```python
from build123d import *

# Parameters (mm, degrees)
SKETCH1_R           = 114.3
SKETCH1_R_2         = 1.778
SKETCH1_W           = 31.75
SKETCH1_H           = 69.85
BOSS_EXTRUDE1_DEPTH = 3.175
SKETCH2_R           = 1.778
SKETCH2_R_2         = 3.914780109
CUT_EXTRUDE1_DEPTH  = 25.4


with BuildPart() as part:
    # Sketch1 → Boss-Extrude1 (new body)
    with BuildSketch(Plane(origin=(0, 0, 0), x_dir=(1, 0, 0), z_dir=(0, 1, 0))):
        Circle(SKETCH1_R)
        with Locations((-14.986, 82.55)):
            Circle(SKETCH1_R_2, mode=Mode.SUBTRACT)
        with Locations((14.986, 82.55)):
            Circle(SKETCH1_R_2, mode=Mode.SUBTRACT)
        with Locations((-14.986, 58.674)):
            Circle(SKETCH1_R_2, mode=Mode.SUBTRACT)
        with Locations((14.986, 58.674)):
            Circle(SKETCH1_R_2, mode=Mode.SUBTRACT)
        with Locations((25.4, 7.874)):
            Circle(SKETCH1_R_2, mode=Mode.SUBTRACT)
        with Locations((25.4, 0)):
            Circle(SKETCH1_R_2, mode=Mode.SUBTRACT)
        with Locations((-25.4, 7.874)):
            Circle(SKETCH1_R_2, mode=Mode.SUBTRACT)
        with Locations((-25.4, 0)):
            Circle(SKETCH1_R_2, mode=Mode.SUBTRACT)
        with Locations((64.389, -15.24)):
            Rectangle(SKETCH1_W, SKETCH1_H, mode=Mode.SUBTRACT)
        with Locations((-64.389, -15.24)):
            Rectangle(SKETCH1_W, SKETCH1_H, mode=Mode.SUBTRACT)
    extrude(amount=BOSS_EXTRUDE1_DEPTH)

    # Sketch2 → Cut-Extrude1 (cut)
    with BuildSketch(Plane(origin=(0, 3.175, 0), x_dir=(1, 0, 0), z_dir=(0, 1, 0))):
        with Locations((-48.514, 32.385)):
            Circle(SKETCH2_R)
        with Locations((48.514, 32.385)):
            Circle(SKETCH2_R)
        with Locations((38.1, 4.739101121)):
            Circle(SKETCH2_R)
        with Locations((-38.1, 4.739101121)):
            Circle(SKETCH2_R)
        with Locations((-38.1, -96.860898879)):
            Circle(SKETCH2_R)
        with Locations((38.1, -96.860898879)):
            Circle(SKETCH2_R)
        with Locations((-38.1, 58.35227567)):
            Circle(SKETCH2_R_2)
        with Locations((38.1, 56.230319403)):
            Circle(SKETCH2_R_2)
        with Locations((80.264, 39.067487207)):
            Circle(SKETCH2_R_2)
        with Locations((-80.264, 39.067487207)):
            Circle(SKETCH2_R_2)
        with BuildLine():
            Line((-25.674625229, -71.132444692), (-25.674625229, -20.989353066))
            ThreePointArc((-25.674625229, -20.989353066), (-19.05, -14.364727837), (-12.425374771, -20.989353066))
            Line((-12.425374771, -20.989353066), (-12.425374771, -71.132444692))
            ThreePointArc((-12.425374771, -71.132444692), (-19.05, -77.757069921), (-25.674625229, -71.132444692))
        make_face()
        with BuildLine():
            Line((12.425374771, -71.132444692), (12.425374771, -20.989353066))
            ThreePointArc((12.425374771, -20.989353066), (19.05, -14.364727837), (25.674625229, -20.989353066))
            Line((25.674625229, -20.989353066), (25.674625229, -71.132444692))
            ThreePointArc((25.674625229, -71.132444692), (19.05, -77.757069921), (12.425374771, -71.132444692))
        make_face()
    extrude(amount=-CUT_EXTRUDE1_DEPTH, mode=Mode.SUBTRACT)


solid = part.part
```
Design review of the part built by this model. Coordinates are the model's own, in mm. A direction names the side the tool comes from. Give positions to 0.01 mm unless a question says otherwise; leave off trailing zeros. Write each loop counter-clockwise with the first axis right and the second up, starting at its lowest first coordinate (ties: lowest second). Pieces come first, ordered by that corner, then holes.
(1) Add section D-D (y = 2.5). Give the number of separate pieces and of enclosed holes in the cut face, and give its area (3 significant figures).
Checked values:
separate pieces: 1
enclosed holes: 22
area: 34,700 mm2
(2) Wall thickness on line 1 along X through (y, z) = (2.7, -14.5); line 2 along Z through (x, y) = (-38.1, 0.6); line 3 along X through (y, z) = (2.6, -57.5): over which ranges is each line inside the solid? List them lowest first.
Checked values:
line 1: x = -113.38 to -80.26, -48.51 to 48.51, 80.26 to 113.38
line 2: z = -107.76 to -62.27, -54.44 to -6.52, -2.96 to 95.08, 98.64 to 107.76
line 3: x = -98.78 to -41.92, -34.28 to -16.32, -13.65 to 13.65, 16.32 to 34.4, 41.8 to 98.78
(3) Add section A-A (z = 74). Give the boundary of the cut face in (x, y) (3 decimals), and give its area (3 significant figures).
Checked values:
outline: (-87.112, 0) - (-25.022, 0) - (-25.022, 3.175) - (-87.112, 3.175) - close; (-13.078, 0) - (13.078, 0) - (13.078, 3.175) - (-13.078, 3.175) - close; (25.022, 0) - (87.112, 0) - (87.112, 3.175) - (25.022, 3.175) - close
area: 477 mm2
(4) Tool access review of faces 1 (the face through (-18.904, 1.61, 77.755)), 2 (the face through (-2, 0, -2)): name each direction out of +Z, -Z, +X, -X, +Y, -Y from which nothing blocks a thin tool from reaching the whole face with its end or side.
Checked values:
face 1: +Y, -Y
face 2: +Z, -Z, +X, -X, -Y
(5) Add section B-B (x = -66). Give the boundary of the cut face in (y, z) (3 decimals).
Checked values:
outline: (0, -93.319) - (3.175, -93.319) - (3.175, -19.685) - (0, -19.685) - close; (0, 50.165) - (3.175, 50.165) - (3.175, 93.319) - (0, 93.319) - close
(6) Mouldability with a two-part tool opening along X and no side actions: class faces 3 (the face through (-2, 3.175, -2)), 4 (the face through (19.196, 1.61, 77.755)), 5 (the face through (39.91, 1.61, -52.76)), 6 (the face through (-114.19, 1.57, -5.03)) as +X half, -X half, draft (parallel to the pull), parting line (faces both ways), or undercut.
Checked values:
face 3: draft
face 4: undercut
face 5: undercut
face 6: parting line
(7) Add section C-C (z = 31). Give the boundary of the cut face in (x, y) (3 decimals).
Checked values:
outline: (-110.016, 0) - (-80.264, 0) - (-80.264, 3.175) - (-110.016, 3.175) - close; (-48.514, 0) - (-25.675, 0) - (-25.675, 3.175) - (-48.514, 3.175) - close; (-12.425, 0) - (12.425, 0) - (12.425, 3.175) - (-12.425, 3.175) - close; (25.675, 0) - (48.514, 0) - (48.514, 3.175) - (25.675, 3.175) - close; (80.264, 0) - (110.016, 0) - (110.016, 3.175) - (80.264, 3.175) - close
(8) Clearance check with flat-ended pins moving along their axes: pin 1 Ø1 at (y, z) = (1, -0.5) entering from -X; pin 2 Ø2 at (x, z) = (-38.1, 96.86) entering from -Y; pin 3 Ø1 at (x, y) = (25.5, 1.5) entering from -Z; pin 4 Ø1.6 at (y, z) = (1, 37.5) entering from -X. State where each tip first meets the part, or that it passes through.
Checked values:
pin 1: stops at x = -114.3
pin 2: passes through
pin 3: stops at z = -111.53
pin 4: stops at x = -108.25
